Here's the drawing with two shaded views (mm, measured from the low corner). I have some questions. Round coordinates to 2 decimals unless told otherwise and drop trailing zeros. Write each loop counter-clockwise with the first axis right and the second up, starting at its lowest first coordinate (ties: lowest second). Pieces come first, ordered by that corner, then holes. Notation, with made-up numbers: (-29.75, 37.5) -> (-10.75, 37.5) arc R21 ccw to (-10.75, 56.5) -> close; hole circle Ø7 at (14.5, 64.5). An arc over 180 degrees is marked (long way). Use CSV: the item, a comma, the result in double quotes.
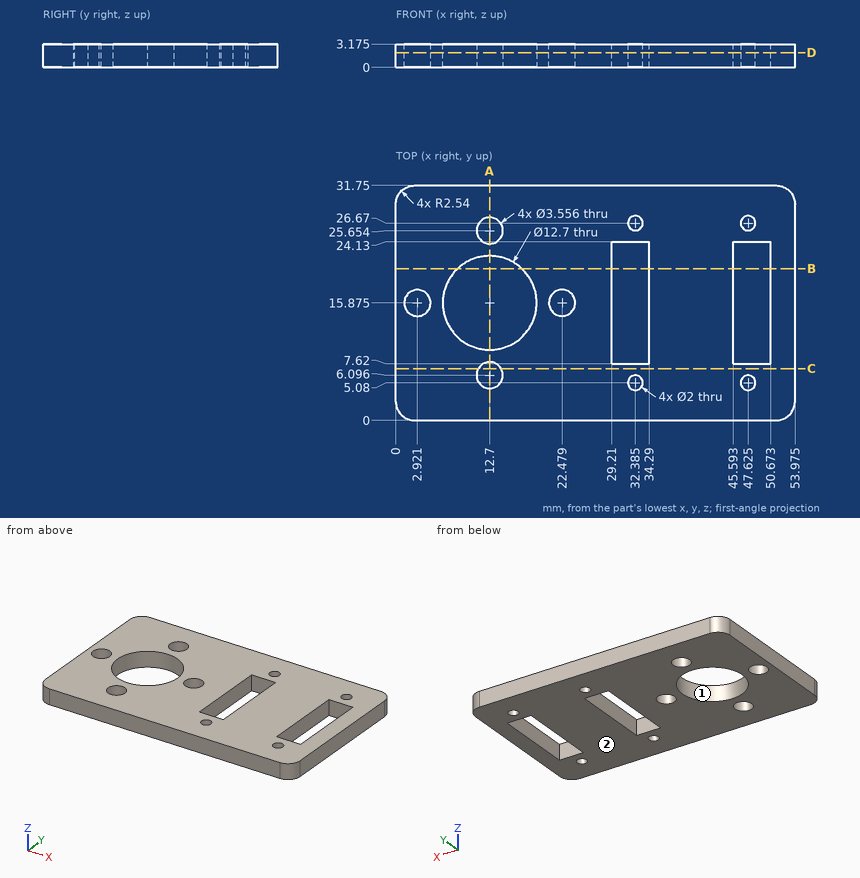
Q1. Please list where these lines run through material, in increasing order: probe 1 along X at (y, z) = (23, 0.4) (3 decimals); probe 2 along Y at (x, z) = (12.7, 1.9) (3 decimals); probe 3 along X at (y, z) = (18, 0.15) (3 decimals).
Resolved:
probe 1,"x = 0 to 29.21, 34.29 to 45.593, 50.673 to 53.975"
probe 2,"y = 0 to 4.318, 7.874 to 9.525, 22.225 to 23.876, 27.432 to 31.75"
probe 3,"x = 0 to 6.716, 18.684 to 29.21, 34.29 to 45.593, 50.673 to 53.975"
Q2. Suppose I cut it at B-B (y = 20.5). Write out the boundary of the cut face in (x, z) (3 decimals).
Resolved:
outline,"(0, 0) -> (8.349, 0) -> (8.349, 3.175) -> (0, 3.175) -> close; (17.051, 0) -> (29.21, 0) -> (29.21, 3.175) -> (17.051, 3.175) -> close; (34.29, 0) -> (45.593, 0) -> (45.593, 3.175) -> (34.29, 3.175) -> close; (50.673, 0) -> (53.975, 0) -> (53.975, 3.175) -> (50.673, 3.175) -> close"
Q3. Suppose I cut it at C-C (y = 7). Write out the boundary of the cut face in (x, z) (3 decimals).
Resolved:
outline,"(0, 0) -> (11.169, 0) -> (11.169, 3.175) -> (0, 3.175) -> close; (14.231, 0) -> (53.975, 0) -> (53.975, 3.175) -> (14.231, 3.175) -> close"
Q4. Suppose I cut it at D-D (z = 2). Count the separate pieces of the cut face and the enclosed holes in it, and give its area (3 significant figures).
Resolved:
separate pieces,"1"
enclosed holes,"11"
area,"1,360 mm^2"
Q5. Suppose I cut it at A-A (x = 12.7). Write out the boundary of the cut face in (y, z) (3 decimals).
Resolved:
outline,"(0, 0) -> (4.318, 0) -> (4.318, 3.175) -> (0, 3.175) -> close; (7.874, 0) -> (9.525, 0) -> (9.525, 3.175) -> (7.874, 3.175) -> close; (22.225, 0) -> (23.876, 0) -> (23.876, 3.175) -> (22.225, 3.175) -> close; (27.432, 0) -> (31.75, 0) -> (31.75, 3.175) -> (27.432, 3.175) -> close"
Q6. If we mould it in two halves opening along X, with no side actions, what happens to the marked faces 1 and 2? For each: released by +X, released by -X, zero draft, split by the parting line, or undercut.
Resolved:
face 1,"undercut"
face 2,"zero draft"
